Geometry check sheet. Reference: the model listing, model coordinates, mm. A direction names the side the tool comes from. Coordinates: 2 decimals unless noted, no trailing zeros. Write each loop counter-clockwise with the first axis right and the second up, starting at its lowest first coordinate (ties: lowest second). Pieces come first, ordered by that corner, then holes. Notation, with made-up numbers: (-19.5, 56) - (37.5, 56) arc R21 cw to (37.5, 91) - close; hole circle Ø11 at (68.25, 28). An arc over 180 degrees is marked (long way). Answer as a JSON object with one key per item and string values. Group by question number.
from build123d import *

# Parameters (mm, degrees)
BOSS_EXTRUDE2_DEPTH = 60
SKETCH3_R           = 4
CUT_EXTRUDE1_DEPTH  = 60
SKETCH4_R           = 6
CUT_EXTRUDE2_DEPTH  = 60
FILLET1_R           = 3
FILLET2_R           = 5
FILLET3_R           = 2


with BuildPart() as part:
    # Sketch1 → Boss-Extrude2 (new body)
    with BuildSketch(Plane.XY):
        Polygon((0, 0), (-52, 0), (-52, -8), (8, -8), (8, 52), (0, 52), align=None)
    extrude(amount=BOSS_EXTRUDE2_DEPTH)

    # Sketch3 → Cut-Extrude1 (cut)
    with BuildSketch(Plane.ZY):
        with Locations(Location((15, 35, 0), (0, 0, 270))):
            Circle(SKETCH3_R)
        with Locations(Location((45, 35, 0), (0, 0, 270))):
            Circle(SKETCH3_R)
    extrude(amount=-CUT_EXTRUDE1_DEPTH, mode=Mode.SUBTRACT)

    # Sketch4 → Cut-Extrude2 (cut)
    with BuildSketch(Plane(origin=(0, 0, 0), x_dir=(1, 0, 0), z_dir=(0, 1, 0))):
        with Locations(Location((-26, -30, 0), (0, 0, 180))):
            Circle(SKETCH4_R)
    extrude(amount=-CUT_EXTRUDE2_DEPTH, mode=Mode.SUBTRACT)

    # Fillet1
    fillet1_edges = [part.edges().sort_by_distance(p)[0] for p in [
        (-52, -4, 60),
        (4, 52, 60),
        (4, 52, 0),
        (-52, -4, 0),
    ]]
    fillet(fillet1_edges, radius=FILLET1_R)

    # Fillet2
    fillet2_edges = [part.edges().sort_by_distance(p)[0] for p in [
        (0, 0, 30),
    ]]
    fillet(fillet2_edges, radius=FILLET2_R)

    # Fillet3
    fillet3_edges = [part.edges().sort_by_distance(p)[0] for p in [
        (8, -8, 30),
    ]]
    fillet(fillet3_edges, radius=FILLET3_R)


solid = part.part
(1) Section check A-A (z = 45). Record the cut outline in (x, y).
(2) Gauge pin test, flat ends, axial feed: pin 1 (3 mm diameter, centred on x = -15.5, z = 25, fed in from +Y); pin 2 (1.5 mm diameter, centred on y = 15, z = 21, fed in from -X). Record the tip position at first contact, or that the pin passes through.
(3) Set-up check for faces 4 (the face through (0.5, 10.1, 0)), 5 (the face through (0, 29, 30)): record each of +Z, -Z, +X, -X, +Y, -Y from which the full face is reachable in a straight line by a thin tool's end or side.
(4) Section check D-D (z = 21). Record the cut outline in (x, y).
(5) Section check B-B (x = -26). Record the cut outline in (y, z), and give its area (3 significant figures).
(6) Draft check along Z on faces 1 (the face through (0.5, 10.1, 60)), 2 (the face through (3.94, 51.1, 0.86)), 3 (the face through (3.9, 38.2, 42.6)). Enter one of: +Z half, -Z half, draft (parallel to the pull), parting line (faces both ways), or undercut.
(7) Material ranges on L1, parallel to Z at x = 6, y = 35; L2, parallel to Z at x = -26, y = -3.25; L3, parallel to X at y = 20.5, z = 46, recorded low to high. Write a range as [from, to].
(8) Section check C-C (y = 35). Record the cut outline in (x, z), and give its area (3 significant figures).
Conclusion:
{
 "1": {"outline": "(-52, -8) - (6, -8) arc R2 ccw to (8, -6) - (8, 31) - (0, 31) - (0, 5) arc R5 cw to (-5, 0) - (-52, 0) - close; (0, 39) - (8, 39) - (8, 52) - (0, 52) - close"},
 "2": {"pin 1": "stops at y = 0", "pin 2": "stops at x = 0"},
 "3": {"face 4": "-Z, +X, -X, +Y, -Y", "face 5": "+Z, -Z, -X, +Y"},
 "4": {"outline": "(-52, -8) - (6, -8) arc R2 ccw to (8, -6) - (8, 52) - (0, 52) - (0, 5) arc R5 cw to (-5, 0) - (-52, 0) - close"},
 "5": {"outline": "(-8, 0) - (0, 0) - (0, 24) - (-8, 24) - close; (-8, 36) - (0, 36) - (0, 60) - (-8, 60) - close", "area": "384 mm^2"},
 "6": {"face 1": "+Z half", "face 2": "-Z half", "face 3": "undercut"},
 "7": {"L1": "z = [0, 11], [19, 41], [49, 60]", "L2": "z = [0, 24], [36, 60]", "L3": "x = [0, 8]"},
 "8": {"outline": "(0, 0) - (8, 0) - (8, 11) - (0, 11) - close; (0, 19) - (8, 19) - (8, 41) - (0, 41) - close; (0, 49) - (8, 49) - (8, 60) - (0, 60) - close", "area": "352 mm^2"}
}
